Autodesk Inventor part; units mm, degrees
ref_plane "YZ Plane" through (0, 0, 0) normal (1, 0, 0) x (0, 1, 0)
ref_plane "XZ Plane" through (0, 0, 0) normal (0, 1, 0) x (-1, 0, 0)
ref_plane "XY Plane" through (0, 0, 0) normal (0, 0, 1) x (1, 0, 0)
sketch "Skizze1" plane through (0, 0, 0) normal (0, 0, 1) x (1, 0, 0)
  spline S0 degree 3 poles (4.1682, 35.1897) (1.1905, 36.4598) (-2.2497, 35.1642) (-6.2549, 34.1582) (-11.7361, 32.1479) (-17.2675, 27.437) (-17.3979, 22.2805) (-19.1794, 11.8373) (-24.2043, -4.2198) (-21.9122, -21.3618) (-15.7263, -32.1361) (-8.9601, -34.8731) (-7.7344, -35.2068) knots 0 0 0 0 0.05535 0.076528 0.211782 0.295547 0.382964 0.432922 0.754884 0.81234 0.967238 1 1 1 1
  spline S1 degree 3 poles (-7.7344, -35.2068) (-2.4391, -36.6482) (4.9342, -35.145) (14.3889, -31.3641) (20.2206, -28.2766) (23.0847, -23.1792) (23.281, -18.9959) (17.3062, -16.4997) (13.7398, -19.2937) (6.9074, -22.9332) (-1.1986, -27.1621) (-10.3055, -22.9326) (-14.0352, -10.4002) (-9.4599, -0.926) (-6.8333, 0.3153) (-5.9182, 2.0588) (-5.9367, 4.1791) (-8.2887, 5.2306) (-8.3641, 10.4373) (-1.0106, 14.1251) (4.0821, 20.0507) (3.0635, 26.3026) (2.9493, 28.6136) (3.7888, 29.834) (5.5778, 31.0924) (6.6132, 32.7745) (5.2458, 34.7086) (4.2657, 35.1481) (4.1682, 35.1897) knots 0 0 0 0 0.14153 0.17035 0.245987 0.25892 0.290227 0.326265 0.372233 0.38898 0.482096 0.508256 0.624416 0.647418 0.715274 0.72607 0.746892 0.801722 0.811885 0.848514 0.916356 0.943374 0.948219 0.962959 0.96651 0.98188 0.998188 1 1 1 1
  arc A0 (-7.9107, 24.207) -> (-7.9109, 20.407) centre (-6.0635, 22.307) ccw
  line L0 (-7.9107, 24.207) -> (-4.2161, 24.2069)
  arc A1 (-4.2163, 20.4069) -> (-4.2161, 24.2069) centre (-6.0635, 22.307) ccw
  line L1 (-4.2163, 20.4069) -> (-7.9109, 20.407)
  spline S2 degree 3 poles (4.1682, 35.1897) (1.1905, 36.4598) (-2.2497, 35.1642) (-6.255, 34.1582) (-11.7361, 32.1479) (-17.2675, 27.437) (-17.3979, 22.2805) (-19.1794, 11.8373) (-24.2043, -4.2198) (-21.9122, -21.3619) (-15.7263, -32.1361) (-8.9601, -34.8731) (-7.7344, -35.2068) knots 0 0 0 0 0.05535 0.076528 0.211782 0.295547 0.382964 0.432922 0.754884 0.81234 0.967238 1 1 1 1
  spline S3 degree 3 poles (-7.7344, -35.2068) (-2.4391, -36.6482) (4.9342, -35.145) (14.3889, -31.3641) (20.2206, -28.2766) (23.0847, -23.1792) (23.281, -18.9959) (17.3062, -16.4997) (13.7398, -19.2937) (6.9074, -22.9332) (-1.1986, -27.1621) (-10.3055, -22.9326) (-14.0352, -10.4002) (-9.4599, -0.926) (-6.8333, 0.3153) (-5.9182, 2.0588) (-5.9367, 4.1791) (-8.2887, 5.2306) (-8.3641, 10.4373) (-1.0106, 14.1251) (4.0821, 20.0507) (3.0635, 26.3026) (2.9493, 28.6136) (3.7888, 29.834) (5.5778, 31.0924) (6.6132, 32.7745) (5.2458, 34.7086) (4.2657, 35.1481) (4.1682, 35.1897) knots 0 0 0 0 0.14153 0.17035 0.245987 0.25892 0.290227 0.326265 0.372233 0.38898 0.482096 0.508256 0.624416 0.647418 0.715274 0.72607 0.746892 0.801722 0.811885 0.848514 0.916356 0.943374 0.948219 0.962959 0.96651 0.98188 0.998188 1 1 1 1
  line L2 (-4.2163, 20.4069) -> (-7.9109, 20.407)
  arc A2 (-4.2163, 20.4069) -> (-4.2161, 24.2069) centre (-6.0635, 22.307) ccw
  line L3 (-7.9107, 24.207) -> (-4.2161, 24.2069)
  arc A3 (-7.9107, 24.207) -> (-7.9109, 20.407) centre (-6.0635, 22.307) ccw
  line L4 (-22.9949, 35.8296) -> (22.9949, 35.8296) construction
  line L5 (22.9949, 35.8296) -> (22.9949, -35.8296) construction
  line L6 (22.9949, -35.8296) -> (-22.9949, -35.8296) construction
  line L7 (-22.9949, -35.8296) -> (-22.9949, 35.8296) construction
  line L8 (-22.9949, 35.8296) -> (22.9949, -35.8296) construction
  line L9 (-22.9949, -35.8296) -> (22.9949, 35.8296) construction
  point P0 (0, 0)
  point P1 (-38.8867, -20.8658)
  point P2 (0, 0)
sketch "Skizze2" plane through (0, 0, 0) normal (0, 0, 1) x (1, 0, 0)
  line L0 (-30, 42.5) -> (30, 42.5)
  line L1 (30, 42.5) -> (30, -42.5)
  line L2 (30, -42.5) -> (-30, -42.5)
  line L3 (-30, -42.5) -> (-30, 42.5)
  line L4 (-30, 42.5) -> (30, -42.5) construction
  line L5 (30, 42.5) -> (-30, -42.5) construction
  arc A0 (-7.9107, 24.207) -> (-7.9109, 20.407) centre (-6.0635, 22.307) ccw
  arc A1 (-7.9107, 24.207) -> (-7.9109, 20.407) centre (-6.0635, 22.307) ccw
  line L6 (-7.9107, 24.207) -> (-4.2161, 24.2069)
  line L7 (-7.9107, 24.207) -> (-4.2161, 24.2069)
  line L8 (-4.2163, 20.4069) -> (-7.9109, 20.407)
  line L9 (-4.2163, 20.4069) -> (-7.9109, 20.407)
  arc A2 (-4.2163, 20.4069) -> (-4.2161, 24.2069) centre (-6.0635, 22.307) ccw
  arc A3 (-4.2163, 20.4069) -> (-4.2161, 24.2069) centre (-6.0635, 22.307) ccw
  line L10 (-22.9949, 35.8296) -> (22.9949, 35.8296) construction
  line L11 (-22.9949, -35.8296) -> (-22.9949, 35.8296) construction
  spline S0 degree 3 poles (4.1682, 35.1897) (1.1905, 36.4598) (-2.2497, 35.1642) (-6.255, 34.1582) (-11.7361, 32.1479) (-17.2675, 27.437) (-17.3979, 22.2805) (-19.1794, 11.8373) (-24.2043, -4.2198) (-21.9122, -21.3619) (-15.7263, -32.1361) (-8.9601, -34.8731) (-7.7344, -35.2068) knots 0 0 0 0 0.05535 0.076528 0.211782 0.295547 0.382964 0.432922 0.754884 0.81234 0.967238 1 1 1 1
  spline S1 degree 3 poles (4.1682, 35.1897) (1.1905, 36.4598) (-2.2497, 35.1642) (-6.2549, 34.1582) (-11.7361, 32.1479) (-17.2675, 27.437) (-17.3979, 22.2805) (-19.1794, 11.8373) (-24.2043, -4.2198) (-21.9122, -21.3618) (-15.7263, -32.1361) (-8.9601, -34.8731) (-7.7344, -35.2068) knots 0 0 0 0 0.05535 0.076528 0.211782 0.295547 0.382964 0.432922 0.754884 0.81234 0.967238 1 1 1 1
  line L12 (-22.9949, 35.8296) -> (22.9949, -35.8296) construction
  line L13 (-22.9949, -35.8296) -> (22.9949, 35.8296) construction
  line L14 (22.9949, -35.8296) -> (-22.9949, -35.8296) construction
  spline S2 degree 3 poles (-7.7344, -35.2068) (-2.4391, -36.6482) (4.9342, -35.145) (14.3889, -31.3641) (20.2206, -28.2766) (23.0847, -23.1792) (23.281, -18.9959) (17.3062, -16.4997) (13.7398, -19.2937) (6.9074, -22.9332) (-1.1986, -27.1621) (-10.3055, -22.9326) (-14.0352, -10.4002) (-9.4599, -0.926) (-6.8333, 0.3153) (-5.9182, 2.0588) (-5.9367, 4.1791) (-8.2887, 5.2306) (-8.3641, 10.4373) (-1.0106, 14.1251) (4.0821, 20.0507) (3.0635, 26.3026) (2.9493, 28.6136) (3.7888, 29.834) (5.5778, 31.0924) (6.6132, 32.7745) (5.2458, 34.7086) (4.2657, 35.1481) (4.1682, 35.1897) knots 0 0 0 0 0.14153 0.17035 0.245987 0.25892 0.290227 0.326265 0.372233 0.38898 0.482096 0.508256 0.624416 0.647418 0.715274 0.72607 0.746892 0.801722 0.811885 0.848514 0.916356 0.943374 0.948219 0.962959 0.96651 0.98188 0.998188 1 1 1 1
  spline S3 degree 3 poles (-7.7344, -35.2068) (-2.4391, -36.6482) (4.9342, -35.145) (14.3889, -31.3641) (20.2206, -28.2766) (23.0847, -23.1792) (23.281, -18.9959) (17.3062, -16.4997) (13.7398, -19.2937) (6.9074, -22.9332) (-1.1986, -27.1621) (-10.3055, -22.9326) (-14.0352, -10.4002) (-9.4599, -0.926) (-6.8333, 0.3153) (-5.9182, 2.0588) (-5.9367, 4.1791) (-8.2887, 5.2306) (-8.3641, 10.4373) (-1.0106, 14.1251) (4.0821, 20.0507) (3.0635, 26.3026) (2.9493, 28.6136) (3.7888, 29.834) (5.5778, 31.0924) (6.6132, 32.7745) (5.2458, 34.7086) (4.2657, 35.1481) (4.1682, 35.1897) knots 0 0 0 0 0.14153 0.17035 0.245987 0.25892 0.290227 0.326265 0.372233 0.38898 0.482096 0.508256 0.624416 0.647418 0.715274 0.72607 0.746892 0.801722 0.811885 0.848514 0.916356 0.943374 0.948219 0.962959 0.96651 0.98188 0.998188 1 1 1 1
  line L15 (22.9949, 35.8296) -> (22.9949, -35.8296) construction
  line L16 (-40, 52.5) -> (40, 52.5)
  line L17 (40, 52.5) -> (40, -52.5)
  line L18 (40, -52.5) -> (-40, -52.5)
  line L19 (-40, -52.5) -> (-40, 52.5)
  line L20 (-40, 52.5) -> (40, -52.5) construction
  line L21 (40, 52.5) -> (-40, -52.5) construction
  point P0 (0, 0)
  point P1 (0, 0)
  point P2 (-38.8867, -20.8658)
  point P3 (0, 0)
  dimension "d0" = 45.9898
  dimension "d1" = 71.6591
  dimension "d2" = 60
  dimension "d3" = 85
  dimension "d4" = 80
  dimension "d5" = 105
extrude "Extrusion1" add sketch "Skizze2" along normal blind 252 contours L16 L17 L18 L19
sketch "Skizze3" plane through (-40, -52.5, 0) normal (0, -1, 0) x (1, 0, 0)
  line L0 (80, 0) -> (0, 0)
  line L1 (10, 0) -> (70, 0)
  line L2 (70, 0) -> (70, 15)
  line L3 (70, 15) -> (10, 15)
  line L4 (10, 15) -> (10, 0)
  line L5 (40, 15) -> (40, 0) construction
  point P0 (40, 0)
  point P1 (70, 0)
  dimension "d8" = 60
  dimension "d9" = 15
extrude "Extrusion2" cut sketch "Skizze3" against normal blind 105
sketch "Skizze4" plane through (0, 0, 0) normal (0, 0, -1) x (-1, 0, 0)
  point P0 (0, 0)
  point P1 (35, -47.5)
  dimension "d12" = 47.5
  dimension "d13" = 35
hole "Bohrung1" at (-35, -47.5, 0) direction (0, 0, 1) diameter 3.242 depth 11.8 tip angle 118
chamfer "Fasen1" distance 1 angle 45 1 edges at (-35, -49.121, 0)
pattern_linear "Rechteckige Anordnung1" count 2 spacing 70 along (1, 0, 0) count 3 spacing 47.5 along (0, 1, 0) of "Bohrung1", "Fasen1"
sketch "Skizze5" plane through (40, -52.5, 0) normal (1, 0, 0) x (0, 0, -1)
  line L0 (0, 105) -> (-252, 105)
  line L1 (-252, 0) -> (-252, 105)
  line L2 (0, 0) -> (0, 105)
  line L3 (0, 0) -> (-252, 0)
  line L4 (-15, 95) -> (-252, 95)
  point P0 (0, 52.5)
  point P1 (-232, 55.1)
  point P2 (-133.5, 55.1)
  point P3 (-35, 55.1)
  point P4 (-252, 52.5)
  dimension "d31" = 20
  dimension "d32" = 118.5
  dimension "d33" = 35
  dimension "d42" = 39.9
hole "Bohrung2" at (40, 2.6, 232) at (40, 2.6, 133.5) at (40, 2.6, 35) direction (-1, 0, 0) diameter 4.5 depth 10 counterbore diameter 8 counterbore depth 4.4
sketch "Skizze6" plane through (-40, 52.5, 0) normal (0, 1, 0) x (1, 0, 0)
  line L0 (80, -129.5) -> (80, -137.5)
  line L1 (80, -228) -> (80, -236)
  line L2 (80, -31) -> (80, -39)
  line L3 (10, -15) -> (10, -252)
  point P0 (40, 0)
  point P1 (80, -232)
  point P2 (34.4, -232)
  point P3 (80, -133.5)
  point P4 (34.4, -133.5)
  point P5 (80, -35)
  point P6 (34.4, -35)
  dimension "d43" = 24.4
hole "Bohrung3" at (-5.6, 52.5, 232) at (-5.6, 52.5, 133.5) at (-5.6, 52.5, 35) direction (0, -1, 0) diameter 4.5 depth 10 tip angle 118 counterbore diameter 8 counterbore depth 4.4
sketch "Skizze7" plane through (-40, -52.5, 0) normal (-1, 0, 0) x (0, 0, 1)
  line L0 (228, 105) -> (236, 105)
  line L1 (129.5, 105) -> (137.5, 105)
  line L2 (31, 105) -> (39, 105)
  line L3 (15, 95) -> (252, 95)
  line L4 (15, 10) -> (252, 10)
  point P0 (0, 52.5)
  point P1 (232, 105)
  point P2 (232, 43)
  point P3 (133.5, 43)
  point P4 (35, 43)
  point P5 (133.5, 105)
  point P6 (35, 105)
  dimension "d67" = 33
hole "Bohrung4" at (-40, -9.5, 232) at (-40, -9.5, 133.5) at (-40, -9.5, 35) direction (1, 0, 0) diameter 4.5 depth 10 tip angle 118 counterbore diameter 8 counterbore depth 4.4
sketch "Skizze8" plane through (30, -52.5, 0) normal (0, -1, 0) x (1, 0, 0)
  circle A0 centre (-35.6, 232) radius 2.25
  circle A1 centre (-35.6, 133.5) radius 2.25
  circle A2 centre (-35.6, 35) radius 2.25
  circle A3 centre (-35.6, 133.5) radius 4
  line L0 (-60, 15) -> (-60, 252)
  point P0 (-30, 0)
  point P1 (-32, 232)
  point P2 (-32, 133.5)
  point P3 (-32, 35)
  point P4 (-34.5692, 20)
  point P5 (-36.6308, 20)
  dimension "d59" = 28
hole "Bohrung5" at (-2, -52.5, 35) at (-2, -52.5, 133.5) at (-2, -52.5, 232) direction (0, 1, 0) diameter 4.5 depth 10 tip angle 118 counterbore diameter 8 counterbore depth 4.4
equation "\"d2\" = Breite_innen"
equation "\"d3\" = Laenge_innen"
equation "\"d4\" = Breite_aussen"
equation "\"d5\" = Laenge_aussen"
equation "\"d6\" = Hoehe_Magazin"
equation "\"d8\" = Breite_innen"
equation "\"d9\" = Ausschubhoehe"
equation "\"d10\" = Laenge_aussen"
equation "\"d26\" = Breite_aussen - Wanddicke"
equation "\"d29\" = -0.5 * Wanddicke + 0.5 * Laenge_aussen"
equation "\"d49\" = Wanddicke"
equation "\"d57\" = Wanddicke"
equation "\"d65\" = Wanddicke"
equation "\"Breite_innen\" = 60"
equation "\"Laenge_innen\" = 85"
equation "\"Breite_aussen\" = Breite_innen + 2 * Wanddicke"
equation "\"Laenge_aussen\" = Laenge_innen + 2 * Wanddicke"
equation "\"Wanddicke\" = 10"
equation "\"Absatz\" = 2"
equation "\"Abstand_Rand\" = 20"
properties part number "TS_V1_Fallmagazin_Wandung_int_CPY"
Geometry check sheet. Reference: the model listing, model coordinates, mm. A direction names the side the tool comes from. Coordinates: 2 decimals unless noted, no trailing zeros. Write each loop counter-clockwise with the first axis right and the second up, starting at its lowest first coordinate (ties: lowest second). Pieces come first, ordered by that corner, then holes. Notation, with made-up numbers: (72.25, 69.5) -> (112.25, 69.5) arc R19 ccw to (112.25, 90.5) -> close; hole circle Ø11 at (47, -38). An arc over 180 degrees is marked (long way). Use CSV: the item, a comma, the result in double quotes. Start each with the question number.
Item 1: Cross-section at C-C, the plane z = 120.5. Record the cut outline in (x, y).
Item 2: Cross-section at B-B, the plane y = 20. Record the cut outline in (x, z), plus the area to 3 significant figures.
Item 3: Set-up check for faces 1 (the flat face through (35.6, 4, 230)), 2 (the cylindrical face through (-1.14, -45.26, 131.42)), 3 (the cylindrical face through (-8.3, 50.27, 32.05)), 4 (the cylindrical face through (-32.761, -11.397, 36.21)), 5 (the flat face through (0, 47, 15)): record each of +Z, -Z, +X, -X, +Y, -Y from which the full face is reachable in a straight line by a thin tool's end or side.
Item 4: Thickness scan on line 1 (Z direction, x = 37, y = 2); line 2 (Y direction, x = 21.5, z = 24); line 3 (X direction, y = 50.2, z = 232). Record the ranges inside material, lowest first.
Item 5: Mould release check, pull along Z, two halves, no side actions. Record for faces 6 (the flat face through (-40, -1, 124)), 7 (the cylindrical face through (37.77, -0.1, 136.45)), 8 (the flat face through (-32, 1, 0)): released by +Z, released by -Z, zero draft, split by the parting line, or undercut.
Item 6: Depth check by flat-ended pin: pin 1 Ø3.5 at (x, y) = (35, 0) entering from -Z; pin 2 Ø5 at (x, z) = (-2, 232) entering from -Y; pin 3 Ø3 at (x, y) = (35, -47.5) entering from -Z. Enter the tip coordinate at first touch or a pass-through.
Item 7: Cross-section at A-A, the plane x = -18. Record the cut outline in (y, z).
Answers:
1,outline,"(-40, -52.5) -> (40, -52.5) -> (40, 52.5) -> (-40, 52.5) -> close; hole (-30, -42.5) -> (30, -42.5) -> (30, 42.5) -> (-30, 42.5) -> close"
2,outline,"(-40, 0) -> (-30, 0) -> (-30, 252) -> (-40, 252) -> close; (30, 0) -> (40, 0) -> (40, 252) -> (30, 252) -> close"
2,area,"5,040 mm^2"
3,face 1,"+X"
3,face 2,"-Y"
3,face 3,"+Y"
3,face 4,"-X"
3,face 5,"-Z, +Y, -Y"
4,line 1,"0 to 31.05, 38.95 to 129.55, 137.45 to 228.05, 235.95 to 252"
4,line 2,"-52.5 to -42.5, 42.5 to 52.5"
4,line 3,"-40 to -9.6, -1.6 to 40"
5,face 6,"zero draft"
5,face 7,"undercut"
5,face 8,"released by -Z"
6,pin 1,"z = 0.87"
6,pin 2,"y = -48.1"
6,pin 3,"z = 11.87"
7,outline,"(-52.5, 15) -> (-42.5, 15) -> (-42.5, 252) -> (-52.5, 252) -> close; (42.5, 15) -> (52.5, 15) -> (52.5, 252) -> (42.5, 252) -> close"
